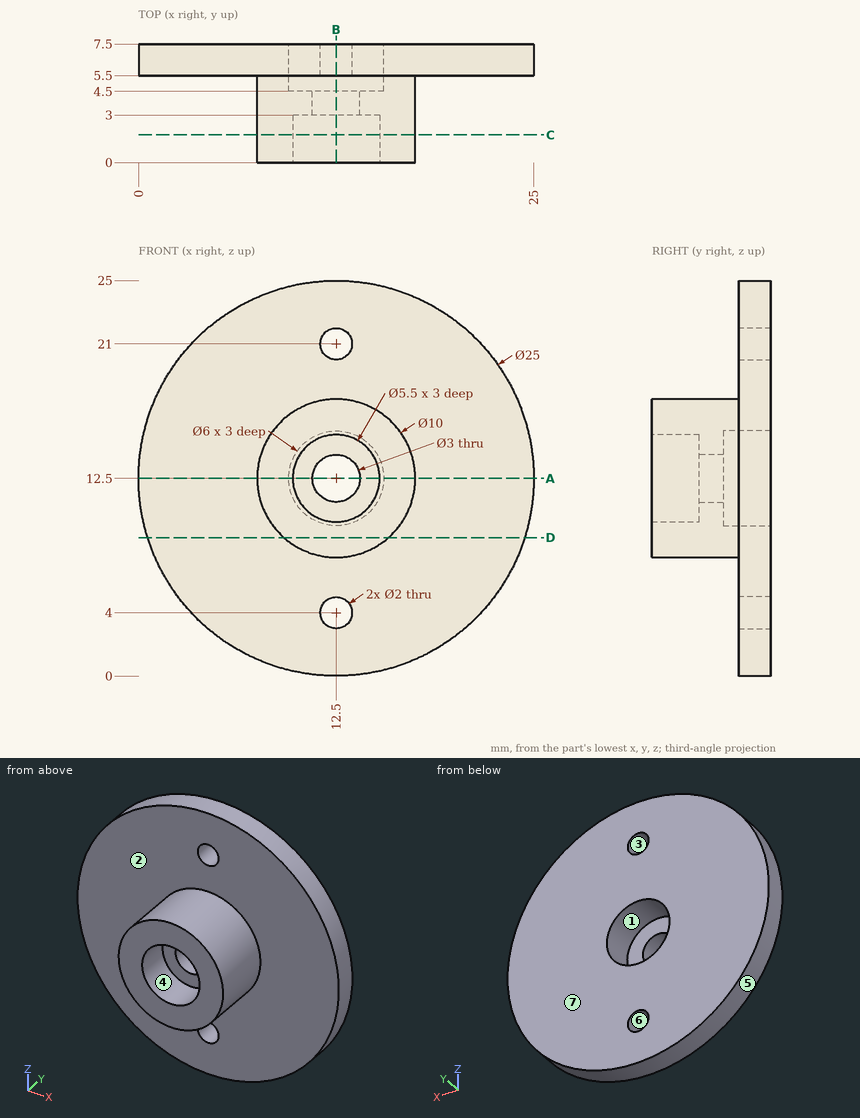
Can you work these out from the drawing? Everything is in mm from the part's minimum corner. A direction names the side the tool comes from. Give positions to 0.01 mm unless a question says otherwise; leave off trailing zeros. Loops run counter-clockwise (first coordinate to the right, second up) from the corner with the lowest first, then second, coordinate; pieces in that order, holes last. Notation, with made-up numbers: (63.5, 24) -> (110.5, 24) arc R18 cw to (110.5, 46) -> close; hole circle Ø10 at (15.25, 84). An arc over 180 degrees is marked (long way). Put each result on its own line as item: value.
(1) Imagine slicing it at D-D on z = 8.75. Write out the boundary of the cut face in (x, y), plus the area to 3 significant figures.
Computed:
outline: (0.58, 5.5) -> (9.19, 5.5) -> (9.19, 0) -> (15.81, 0) -> (15.81, 5.5) -> (24.42, 5.5) -> (24.42, 7.5) -> (0.58, 7.5) -> close
area: 84.1 mm^2
(2) Imagine slicing it at A-A on z = 12.5. Write out the boundary of the cut face in (x, y), plus the area to 3 significant figures.
Computed:
outline: (0, 5.5) -> (7.5, 5.5) -> (7.5, 0) -> (9.75, 0) -> (9.75, 3) -> (11, 3) -> (11, 4.5) -> (9.5, 4.5) -> (9.5, 7.5) -> (0, 7.5) -> close; (14, 3) -> (15.25, 3) -> (15.25, 0) -> (17.5, 0) -> (17.5, 5.5) -> (25, 5.5) -> (25, 7.5) -> (15.5, 7.5) -> (15.5, 4.5) -> (14, 4.5) -> close
area: 66.0 mm^2
(3) For the marked faces 1, 2 and 3, which set-ups out of +Z, -Z, +X, -X, +Y, -Y let a thin tool reach every point of the face, with its end or its side?
Computed:
face 1: +Y
face 2: -Y
face 3: +Y, -Y
(4) I'm going to push flat-ended pins straight in: pin 1 Ø5 at (x, z) = (12.5, 12.5) entering from +Y; pin 2 Ø4.5 at (x, z) = (12.5, 12.5) entering from -Y; pin 3 Ø6.5 at (x, z) = (12.5, 11.5) entering from +Y; pin 4 Ø3 at (y, z) = (2.5, 8.5) entering from -X. Where does each tip first touch, or does it pass through?
Computed:
pin 1: y = 4.5
pin 2: y = 3
pin 3: y = 7.5
pin 4: x = 8.17
(5) Please list where these lines run through material, in increasing order: probe 1 along X at (y, z) = (3.65, 12.5); probe 2 along Y at (x, z) = (2.5, 18.75); probe 3 along X at (y, z) = (0.5, 16.5). Write a range as [from, to].
Computed:
probe 1: [7.5, 11], [14, 17.5]
probe 2: [5.5, 7.5]
probe 3: [9.5, 15.5]
(6) Thinking about a two-plate mould opening in Z: for the marked faces 4, 5, 6 and 7, which applies, pulls with the +Z half, pulls with the -Z half, needs draft (parallel to the pull), parting line crosses it, or undercut?
Computed:
face 4: undercut
face 5: parting line crosses it
face 6: undercut
face 7: needs draft
(7) Imagine slicing it at B-B on x = 12.5. Write out the boundary of the cut face in (y, z).
Computed:
outline: (0, 7.5) -> (5.5, 7.5) -> (5.5, 5) -> (7.5, 5) -> (7.5, 9.5) -> (4.5, 9.5) -> (4.5, 11) -> (3, 11) -> (3, 9.75) -> (0, 9.75) -> close; (0, 15.25) -> (3, 15.25) -> (3, 14) -> (4.5, 14) -> (4.5, 15.5) -> (7.5, 15.5) -> (7.5, 20) -> (5.5, 20) -> (5.5, 17.5) -> (0, 17.5) -> close; (5.5, 0) -> (7.5, 0) -> (7.5, 3) -> (5.5, 3) -> close; (5.5, 22) -> (7.5, 22) -> (7.5, 25) -> (5.5, 25) -> close
(8) Imagine slicing it at C-C on y = 1.75. Write out the boundary of the cut face in (x, z), plus the area to 3 significant figures.
Computed:
outline: circle Ø10 at (12.5, 12.5); hole circle Ø5.5 at (12.5, 12.5)
area: 54.8 mm^2
